```python
from build123d import *

# Parameters (mm, degrees)
CYLINDER003_R     = 5.8928
CYLINDER003_DEPTH = 2.032
SKETCH003_W       = 19.05
SKETCH003_H       = 30.48
PAD_DEPTH         = 3.048
PAD001_DEPTH      = 19.05
SKETCH005_W       = 4.7498
SKETCH005_H       = 3.048
PAD002_DEPTH      = 6.35


with BuildPart() as part:
    # Cylinder003 → Cylinder003 (new body)
    with BuildSketch(Plane(origin=(0, -38.1, 34.923527), x_dir=(1, 0, 0), z_dir=(0, 0, 1))):
        Circle(CYLINDER003_R)
    extrude(amount=CYLINDER003_DEPTH)

    # Sketch003 → Pad (new body)
    with BuildSketch(Plane(origin=(0, -38.1, 36.955527), x_dir=(1, 0, 0), z_dir=(0, 0, 1))):
        Rectangle(SKETCH003_W, SKETCH003_H)
    extrude(amount=PAD_DEPTH)

    # Sketch004 → Pad001 (new body)
    with BuildSketch(Plane(origin=(-9.525, -38.1, 34.923527), x_dir=(0, -1, 0), z_dir=(-1, 0, 0))):
        Polygon((-15.24, 5.08), (-27.812359, 17.652359), (-65.912359, 17.652359), (-65.912359, 14.604359), (-27.812359, 14.604359), (-15.24, 2.032), align=None)
    extrude(amount=-PAD001_DEPTH)

    # Sketch005 → Pad002 (new body)
    with BuildSketch(Plane(origin=(0, -38.1, 36.955527), x_dir=(1, 0, 0), z_dir=(0, 0, -1))):
        with Locations((-2.0701, 13.716)):
            Rectangle(SKETCH005_W, SKETCH005_H)
    extrude(amount=PAD002_DEPTH)


solid = part.part
```
Check sheet for the modelled part. Datum: model origin and axes. Units: mm. A direction names the side the tool comes from. Coordinates: 2 decimals unless noted, no trailing zeros. Write each loop counter-clockwise with the first axis right and the second up, starting at its lowest first coordinate (ties: lowest second). Pieces come first, ordered by that corner, then holes. Notation, with made-up numbers: M 57,36.5 L 92,36.5 A17 cw 92,61.5 Z; hole C 37.5,79 d8. An arc over 180 degrees is marked long. Write item = value, one per line. Start each with the question number.
1. Tool access check on faces 1 (the flat face through (0, -38, 34.924)), 2 (the flat face through (-4.445, -52, 34)), 3 (the flat face through (0, -38, 40.004)), 4 (the flat face through (0.305, -52, 34)). Record the directions out of +Z, -Z, +X, -X, +Y, -Y that give a thin tool (end or side, any length) a straight path to the whole face; none if there is none.
2. Thickness scan on probe 1 along Z at (x, y) = (5, -7); probe 2 along Z at (x, y) = (-1.25, -24); probe 3 along Y at (x, z) = (0.75, 40.25). Record the ranges inside material, lowest first.
3. Sectioned sample at D-D (y = 21). Record the cut outline in (x, z) (3 decimals).
4. Sectioned sample at A-A (x = 7.5). Record the cut outline in (y, z), then the cut area to 3 significant figures.
5. Sectioned sample at C-C (x = 4). Record the cut outline in (y, z).
6. Sectioned sample at B-B (y = -38.1). Record the cut outline in (x, z) (3 decimals).
7. Go/stop test with flat-tipped pins: pin 1 (9.5 mm diameter, centred on x = 1, y = -40.5, fed in from -Z); pin 2 (2.5 mm diameter, centred on y = -51.5, z = 34.5, fed in from -X) (3 decimals); pin 3 (5 mm diameter, centred on x = -2.5, z = 33.5, fed in from +Y). Record where each tip stops, or that it passes through.
The answers:
q1.face_1 = -Z, +X, -X, +Y
q1.face_2 = -Z, -X, -Y
q1.face_3 = +Z, +X, -X, -Y
q1.face_4 = -Z, +X, -Y
q2.probe_1 = 49.53 to 52.58
q2.probe_2 = 36.96 to 40
q2.probe_3 = -22.61 to -19.57
q3.outline = M -9.525,49.528 L 9.525,49.528 L 9.525,52.576 L -9.525,52.576 Z
q4.outline = M -53.34,36.96 L -22.86,36.96 L -10.29,49.53 L 27.81,49.53 L 27.81,52.58 L -10.29,52.58 L -22.86,40 L -53.34,40 Z
q4.area = 247 mm²
q5.outline = M -53.34,36.96 L -42.43,36.96 L -42.43,34.92 L -33.77,34.92 L -33.77,36.96 L -22.86,36.96 L -10.29,49.53 L 27.81,49.53 L 27.81,52.58 L -10.29,52.58 L -22.86,40 L -53.34,40 Z
q6.outline = M -9.525,36.956 L -5.893,36.956 L -5.893,34.924 L 5.893,34.924 L 5.893,36.956 L 9.525,36.956 L 9.525,40.004 L -9.525,40.004 Z
q7.pin_1 = 34.92
q7.pin_2 = -4.445
q7.pin_3 = -32.22
